For this review, take the finished solid that the model builds, in its own axes (mm). Face numbers are marked on the shaded views. A direction names the side the tool comes from. Coordinates: 2 decimals unless noted, no trailing zeros. Loops run counter-clockwise (first coordinate to the right, second up) from the corner with the lowest first, then second, coordinate; pieces in that order, holes last. Notation, with made-up numbers: (-26, -21.75) - (33, -21.75) arc R14 cw to (33, 4.25) - close; hole circle Ø1 at (30, 67.25). An arc over 180 degrees is marked (long way). Answer as a JSON object with one key per item and string values. Group by question number.
Item 1: We need section C-C (x = 1.5). Give the boundary of the cut face in (y, z) (1 decimal).
Item 2: Tool access review of the marked faces 1 and 2: name each direction out of +Z, -Z, +X, -X, +Y, -Y from which nothing blocks a thin tool from reaching the whole face with its end or side.
Item 3: We need section B-B (x = -14). Give the boundary of the cut face in (y, z) (1 decimal).
Item 4: Clearance check with flat-ended pins moving along their axes: pin 1 (2.5 mm diameter, centred on x = -33.02, z = -15.875, fed in from +Y); pin 2 (9 mm diameter, centred on x = -13.86, z = 10.79, fed in from -Y); pin 3 (2.5 mm diameter, centred on x = 34, z = 15.5, fed in from -Y) (3 decimals). State where each tip first meets the part, or that it passes through.
Item 5: We need section A-A (y = 5.5). State how many separate pieces and enclosed holes the cut face has, then the cut area to 3 significant figures.
Item 6: Mouldability with a two-part tool opening along X and no side actions: class the marked faces 3, 4 and 5 as released by +X, released by -X, zero draft, split by the parting line, or undercut.
Item 7: To check wall thickness, follow line 1 (Z direction, x = 33.02, y = 7); line 2 (Z direction, x = -9, y = 2); line 3 (Z direction, x = 0.5, y = 7.25). State the ranges of each line that lie inside material, in increasing order.
from build123d import *

# Parameters (mm, degrees)
SKETCH1_W               = 76.2
SKETCH1_H               = 50.8
BOSS_EXTRUDE1_DEPTH     = 9.525
F_1_4_CLEARANCE_HOLE1_D = 6.7564
CUT_EXTRUDE1_DEPTH      = 65.210401221
SKETCH5_R               = 2.38125
CUT_EXTRUDE2_DEPTH      = 47.770670564
F_8_CLEARANCE_HOLE1_D   = 4.4958
CUT_EXTRUDE3_DEPTH      = 4.7625
CUT_EXTRUDE4_DEPTH      = 3.175
SKETCH11_R              = 3.175
CUT_EXTRUDE5_DEPTH      = 6.35


with BuildPart() as part:
    # Sketch1 → Boss-Extrude1 (new body)
    with BuildSketch(Plane(origin=(0, 0, 0), x_dir=(1, 0, 0), z_dir=(0, 1, 0))):
        Rectangle(SKETCH1_W, SKETCH1_H)
    extrude(amount=BOSS_EXTRUDE1_DEPTH)

    # 1/4 Clearance Hole1 (through all)
    with Locations(Plane(origin=(0, 9.525, 0), x_dir=(1, 0, 0), z_dir=(0, 1, 0))):
        with Locations((0, 14.61008), (-13.86078, -10.78992), (13.86078, -10.78992)):
            Hole(F_1_4_CLEARANCE_HOLE1_D / 2)

    # Sketch4 → Cut-Extrude1 (cut, through all)
    with BuildSketch(Plane.XY.offset(25.4)):
        with BuildLine():
            Line((-27.6225, 9.525), (-18.0975, 9.525))
            ThreePointArc((-18.0975, 9.525), (-22.86, 4.7625), (-27.6225, 9.525))
        make_face()
        with BuildLine():
            Line((18.0975, 9.525), (27.6225, 9.525))
            ThreePointArc((27.6225, 9.525), (22.86, 4.7625), (18.0975, 9.525))
        make_face()
    extrude(amount=-CUT_EXTRUDE1_DEPTH, mode=Mode.SUBTRACT)

    # Sketch5 → Cut-Extrude2 (cut, through all)
    with BuildSketch(Plane(origin=(0, 9.525, 0), x_dir=(1, 0, 0), z_dir=(0, 1, 0))):
        with Locations(Location((0, -3.175, 0), (0, 0, 270))):
            Circle(SKETCH5_R)
    extrude(amount=-CUT_EXTRUDE2_DEPTH, mode=Mode.SUBTRACT)

    # #8 Clearance Hole1 (through all)
    with Locations(Plane(origin=(0, 9.525, 0), x_dir=(1, 0, 0), z_dir=(0, 1, 0))):
        with Locations((-33.02, 15.875), (-33.02, -15.875), (33.02, -15.875), (33.02, 15.875), (-12.7, 15.875), (12.7, 15.875), (0, -15.875)):
            Hole(F_8_CLEARANCE_HOLE1_D / 2)

    # Sketch8 → Cut-Extrude3 (cut)
    with BuildSketch(Plane.XZ):
        Polygon((-17.28978, 4.82092), (-10.43178, 4.82092), (-7.00278, 10.760122219), (-10.43178, 16.699324438), (-17.28978, 16.699324438), (-20.71878, 10.760122219), align=None)
        Polygon((10.43178, 4.82092), (17.28978, 4.82092), (20.71878, 10.760122219), (17.28978, 16.699324438), (10.43178, 16.699324438), (7.00278, 10.760122219), align=None)
        Polygon((-3.429, -20.57908), (3.429, -20.57908), (6.858, -14.639877781), (3.429, -8.700675562), (-3.429, -8.700675562), (-6.858, -14.639877781), align=None)
    extrude(amount=-CUT_EXTRUDE3_DEPTH, mode=Mode.SUBTRACT)

    # Sketch9 → Cut-Extrude4 (cut)
    with BuildSketch(Plane.XZ):
        Polygon((-37.465, 13.308678053), (-37.465, 18.441321947), (-33.02, 21.007643893), (-28.575, 18.441321947), (-28.575, 13.308678053), (-33.02, 10.742356107), align=None)
        Polygon((-4.445, 13.308678053), (-4.445, 18.441321947), (0, 21.007643893), (4.445, 18.441321947), (4.445, 13.308678053), (0, 10.742356107), align=None)
        Polygon((28.575, 13.308678053), (28.575, 18.441321947), (33.02, 21.007643893), (37.465, 18.441321947), (37.465, 13.308678053), (33.02, 10.742356107), align=None)
        Polygon((28.575, -18.441321947), (28.575, -13.308678053), (33.02, -10.742356107), (37.465, -13.308678053), (37.465, -18.441321947), (33.02, -21.007643893), align=None)
        Polygon((8.255, -18.441321947), (8.255, -13.308678053), (12.7, -10.742356107), (17.145, -13.308678053), (17.145, -18.441321947), (12.7, -21.007643893), align=None)
        Polygon((-17.145, -18.441321947), (-17.145, -13.308678053), (-12.7, -10.742356107), (-8.255, -13.308678053), (-8.255, -18.441321947), (-12.7, -21.007643893), align=None)
        Polygon((-37.465, -18.441321947), (-37.465, -13.308678053), (-33.02, -10.742356107), (-28.575, -13.308678053), (-28.575, -18.441321947), (-33.02, -21.007643893), align=None)
    extrude(amount=-CUT_EXTRUDE4_DEPTH, mode=Mode.SUBTRACT)

    # Sketch11 → Cut-Extrude5 (cut)
    with BuildSketch(Plane(origin=(0, 9.525, 0), x_dir=(1, 0, 0), z_dir=(0, 1, 0))):
        with Locations(Location((0, -3.175, 0), (0, 0, 270))):
            Circle(SKETCH11_R)
    extrude(amount=-CUT_EXTRUDE5_DEPTH, mode=Mode.SUBTRACT)


solid = part.part
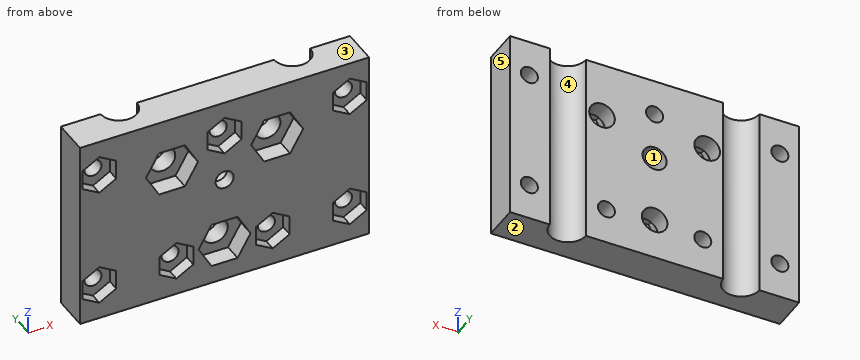
Check sheet entries:
{
 "1": {"outline": "(0, -25.4) - (9.5, -25.4) - (9.5, -17.6) - (4.8, -17.6) - (4.8, -20.6) - (0, -20.6) - close; (0, -8.7) - (4.8, -8.7) - (4.8, -11.6) - (9.5, -11.6) - (9.5, 0.4) - (3.2, 0.4) - (3.2, 1.3) - (0, 1.3) - close; (0, 5) - (3.2, 5) - (3.2, 6) - (9.5, 6) - (9.5, 14.2) - (3.2, 14.2) - (3.2, 11.6) - (0, 11.6) - close; (0, 20.1) - (3.2, 20.1) - (3.2, 17.5) - (9.5, 17.5) - (9.5, 25.4) - (0, 25.4) - close"},
 "2": {"face 1": "+Y", "face 2": "-Z, +X, -X, +Y, -Y"},
 "3": {"outline": "(0, -25.4) - (9.5, -25.4) - (9.5, -17.7) - (3.2, -17.7) - (3.2, -20.3) - (0, -20.3) - close; (0, -11.5) - (3.2, -11.5) - (3.2, -14) - (9.5, -14) - (9.5, 7.4) - (4.8, 7.4) - (4.8, 4.8) - (0, 4.8) - close; (0, 16.7) - (4.8, 16.7) - (4.8, 14.2) - (9.5, 14.2) - (9.5, 25.4) - (0, 25.4) - close"},
 "4": {"pin 1": "passes through", "pin 2": "stops at y = 4.76", "pin 3": "stops at y = 3.175"},
 "5": {"separate pieces": "3", "enclosed holes": "11", "area": "3,100 mm2"},
 "6": {"face 3": "zero draft", "face 4": "undercut", "face 5": "released by +X"},
 "7": {"line 1": "z = -25.4 to -18.12, -13.63 to 13.63, 18.12 to 25.4", "line 2": "z = -25.4 to -18.87, -12.88 to 7.3, 14.22 to 25.4", "line 3": "z = -25.4 to -17.95, -11.27 to 0.04, 6.31 to 13.68, 18.07 to 25.4"}
}
